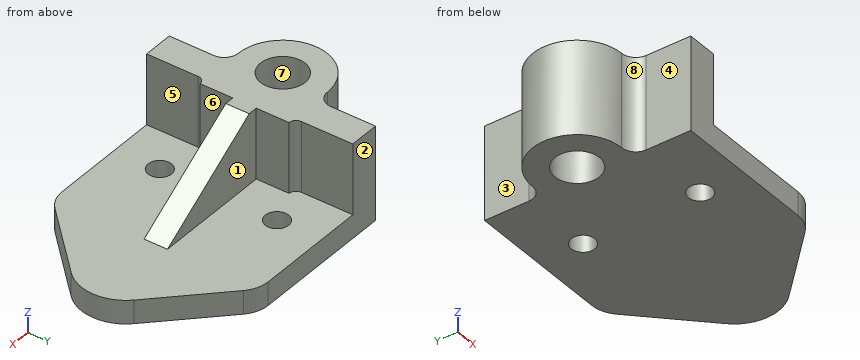
Autodesk Fusion 360 part; units mm, degrees
sketch "base" plane through (0, 0, 0) normal (0, 0, 1) x (1, 0, 0)
  line L0 (75, -35) -> (136.6142, -35)
  line L1 (142, -35) -> (142, 53)
  line L2 (136.6142, 53) -> (75, 53)
  line L3 (75, 53) -> (75, -35)
  line L4 (142, 9) -> (142, 14)
  line L5 (142, 9) -> (142, 4)
  line L6 (136.6142, 53) -> (106, 53)
  line L7 (142, 9) -> (142, 34)
  circle A0 centre (106, 34) radius 5
  line L8 (142, 9) -> (75, 9) construction
  circle A1 centre (106, -16) radius 5
  line L9 (145.8078, -31.1912) -> (172.5588, -4.4333)
  line L10 (172.5588, 22.4333) -> (145.8078, 49.1912)
  arc A2 (172.5588, -4.4333) -> (172.5588, 22.4333) centre (159.122, 9) ccw
  arc A3 (136.6142, -35) -> (145.8078, -31.1912) centre (136.6142, -22) ccw
  arc A4 (145.8078, 49.1912) -> (136.6142, 53) centre (136.6142, 40) ccw
  dimension "d1" = 67
  dimension "d2" = 88
  dimension "d3" = 5
  dimension "d4" = 5
  dimension "d5" = 36
  dimension "d6" = 25
  dimension "d7" = 10
  dimension "d8" = 19
  dimension "d9" = 13
  dimension "d10" = 13
extrude "Extrude1" add sketch "base" along normal blind 10
sketch "top" plane through (0, 0, 10) normal (0, 0, 1) x (-1, 0, 0)
  circle A0 centre (-106, 16) radius 5
  circle A1 centre (-106, -34) radius 5
  arc A2 (-145.8078, -49.1912) -> (-136.6142, -53) centre (-136.6142, -40) ccw
  line L0 (-136.6142, -53) -> (-75, -53)
  line L1 (-75, -53) -> (-75, 35)
  line L2 (-75, 35) -> (-136.6142, 35)
  arc A3 (-136.6142, 35) -> (-145.8078, 31.1912) centre (-136.6142, 22) ccw
  line L3 (-145.8078, 31.1912) -> (-172.5588, 4.4333)
  arc A4 (-172.5588, 4.4333) -> (-172.5588, -22.4333) centre (-159.122, -9) ccw
  line L4 (-172.5588, -22.4333) -> (-145.8078, -49.1912)
  line L5 (-75, -53) -> (-88, -53)
  circle A5 centre (-69, -9) radius 9.5
  line L6 (-142, -14) -> (-95, -14)
  line L7 (-142, -14) -> (-142, -4)
  line L8 (-142, -4) -> (-95, -4)
  line L9 (-95, -4) -> (-95, -14)
  line L10 (-91, -9) -> (-91, -28)
  line L11 (-91, -28) -> (-91, -9)
  line L12 (-91, -9) -> (-91, 10)
  line L13 (-91, -28) -> (-91, -28)
  line L14 (-88, -31) -> (-88, -53)
  line L15 (-91, 10) -> (-91, 10)
  line L16 (-88, 13) -> (-88, 35)
  arc A6 (-88, -31) -> (-91, -28) centre (-91, -31) ccw
  arc A7 (-91, 10) -> (-88, 13) centre (-91, 13) ccw
  line L17 (-95, -14) -> (-91, -14)
  line L18 (-91, -4) -> (-95, -4)
  line L19 (-75, -53) -> (-75, -34)
  line L20 (-88, 35) -> (-75, 35)
  line L21 (-75, 35) -> (-75, 16)
  line L22 (-69, -28) -> (-69, -28)
  arc A8 (-69, -28) -> (-75, -34) centre (-69, -34) ccw
  line L23 (-69, 10) -> (-69, 10)
  arc A9 (-75, 16) -> (-69, 10) centre (-69, 16) ccw
  arc A10 (-69, -28) -> (-69, 10) centre (-69, -9) ccw
  dimension "d13" = 19
  dimension "d14" = 3
  dimension "d15" = 3
  dimension "d16" = 6
  dimension "d17" = 6
extrude "Extrude2" add sketch "top" against normal blind 10 contours L1 A5 A8 A9 A10
extrude "Extrude3" add sketch "top" along normal blind 30 contours L6 L7 L8 L9
sketch "ramp" plane through (0, 4, 0) normal (0, -1, 0) x (1, 0, 0)
  line L0 (95, 10) -> (142, 10)
  line L1 (142, 10) -> (142, 40)
  line L2 (142, 40) -> (95, 40)
  line L3 (95, 40) -> (95, 10)
  line L4 (95, 40) -> (142, 10)
  line L5 (142, 10) -> (142, 40)
  line L6 (95, 40) -> (142, 40)
extrude "Extrude4" cut sketch "ramp" against normal blind 10 contours L1 L2 L4 L5 L6
extrude "Extrude5" add sketch "top" along normal blind 30 contours L9 L10 L11 L12 L17 L18
extrude "Extrude6" add sketch "top" along normal blind 30 contours L0 L1 L2 L5 A5 L10 L11 L12 L14 L16 A6 A7 L19 L20 L21
extrude "Extrude7" add sketch "top" along normal blind 30 contours L1 A5 A8 A9 A10
extrude "Extrude8" cut 1 faces at (75.8602, 7.6409, 10) along direction (0, 0, -1) blind 10
The listing builds one solid part. Answer for the finished solid, in the listing's coordinates (mm). Face numbers are marked on the shaded views. A direction names the side the tool comes from. Round coordinates to 2 decimals unless told otherwise and drop trailing zeros. Order: outer loops, then holes, each group sorted by start corner. A loop starts at its lowest first (then second) coordinate and runs counter-clockwise, first axis right, second up. Notation, with made-up numbers: M 63.25,29 L 96.25,29 A8 ccw 96.25,37 Z; hole C 16,-19.75 d3. An arc over 180 degrees is marked long. Answer in a Markdown table with one row per item. Add a question column.
1) Determine the mould class of the marked faces 6, 7 and 8 for opening direction Y: pulls with the +Y half, pulls with the -Y half, needs draft (parallel to the pull), parting line crosses it, or undercut.
2) The part is cut by section B-B on y = -14.5. Determine the outline of the cut face in (x, z).
3) The part is cut by section C-C on x = 115.5. Determine the outline of the cut face in (y, z).
4) Which of the six approach directions +Z, -Z, +X, -X, +Y, -Y give full straight-line access (tool end or side, diameter ignored) to the marked faces 1, 2, 3, 4 and 5?
5) Consider line 1 along Y through (x, z) = (69, 31); line 2 along Z through (x, y) = (149.5, -18.5); line 3 along X through (y, z) = (47, 36). Determine where each line is inside the solid, lowest interval first. Write a range as from..to.
6) The part is cut by section A-A on z = 22. Determine the outline of the cut face in (x, y), plus the area to 3 significant figures.
7) Flat-ended cylindrical pins translate along their axes: pin 1 Ø9.5 at (y, z) = (-25.5, 17) entering from -X; pin 2 Ø11 at (y, z) = (40, 27) entering from +X; pin 3 Ø9 at (x, z) = (119.5, 18) entering from -Y. Find the tip coordinate at first contact, or state that the pin passes through.
8) The part is cut by section D-D on y = 42.5. Determine the outline of the cut face in (x, z), plus the area to 3 significant figures.
Findings below:
| question | item | result |
|---|---|---|
| 1 | face 6 | needs draft |
| 1 | face 7 | undercut |
| 1 | face 8 | pulls with the -Y half |
| 2 | outline | M 74.81,0 L 101.23,0 L 101.23,10 L 88,10 L 88,40 L 74.81,40 Z; M 110.77,0 L 162.49,0 L 162.49,10 L 110.77,10 Z |
| 3 | outline | M -35,0 L 53,0 L 53,10 L 14,10 L 14,26.91 L 4,26.91 L 4,10 L -35,10 Z |
| 4 | face 1 | +Z, +X, +Y |
| 4 | face 2 | +Z, -Z, +X, -X, +Y |
| 4 | face 3 | +Z, -Z, -X, +Y |
| 4 | face 4 | +Z, -Z, -X, -Y |
| 4 | face 5 | +Z, +X, -Y |
| 5 | line 1 | y = -10..-0.5, 18.5..28 |
| 5 | line 2 | z = 0..10 |
| 5 | line 3 | x = 75..88 |
| 6 | outline | M 69,-10 A6 cw 75,-16 L 75,-35 L 88,-35 L 88,-13 A3 cw 91,-10 L 91,4 L 123.2,4 L 123.2,14 L 91,14 L 91,28 A3 cw 88,31 L 88,53 L 75,53 L 75,34 A6 cw 69,28 A19 ccw Z; hole C 69,9 d19 |
| 6 | area | 2,110 mm² |
| 7 | pin 1 | stops at x = 75 |
| 7 | pin 2 | stops at x = 88 |
| 7 | pin 3 | stops at y = 4 |
| 8 | outline | M 75,0 L 152.5,0 L 152.5,10 L 88,10 L 88,40 L 75,40 Z |
| 8 | area | 1,160 mm² |
